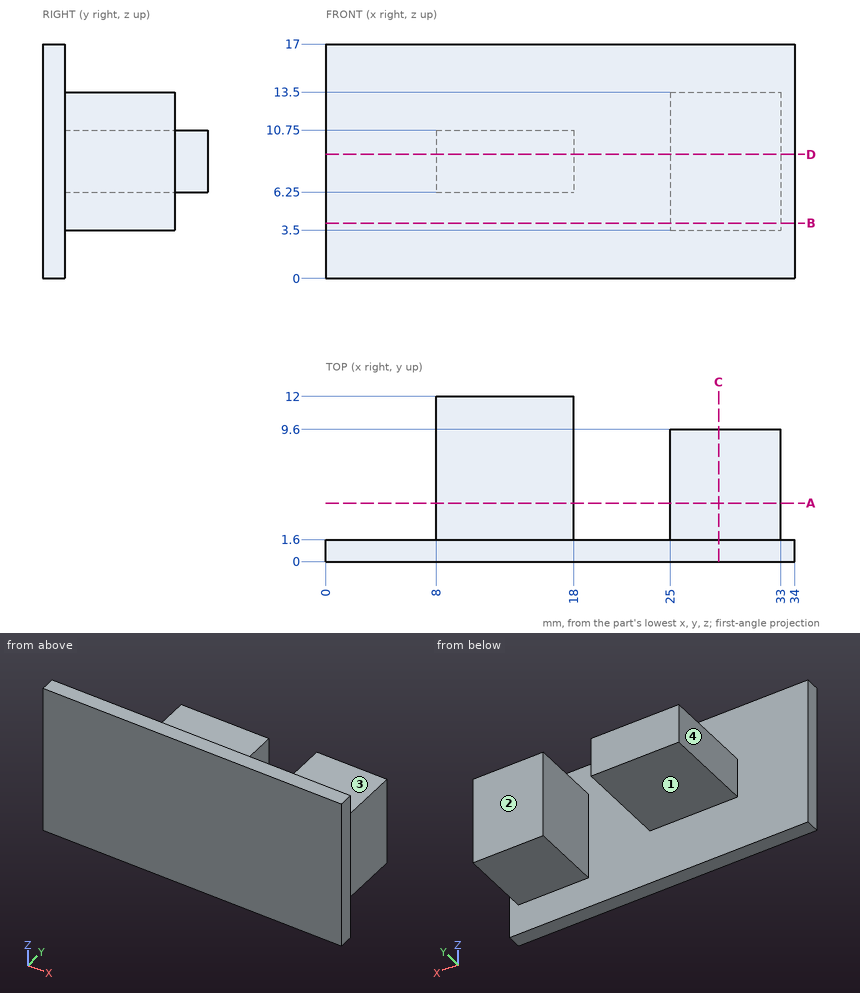
Answer from the drawing. Dimensions are ordinates in mm from the lowest x, y and z of the part. A direction names the side the tool comes from. Round coordinates to 2 decimals unless told otherwise and drop trailing zeros. Loops run counter-clockwise (first coordinate to the right, second up) from the corner with the lowest first, then second, coordinate; pieces in that order, holes last.
1) For the marked faces 1, 2, 3 and 4, determine the directions among +Z, -Z, +X, -X, +Y, -Y from which every point of the face is accessible in a straight line to the end or side of a thin tool.
Outcome:
face 1: -Z, -X, +Y
face 2: +Z, -Z, +X, +Y
face 3: +Z, +X, -X, +Y
face 4: +Z, -Z, -X, +Y
2) Given P1, Ø3.5, axis at y = 7, z = 8.5, coming from the -X side; P2, Ø3, axis at x = 12.5, z = 9, coming from the -Y side; P3, Ø6, axis at x = 4, y = 10, coming from the -Z side; P4, Ø6, axis at y = 7.5, z = 6, coming from the +X side, each flat-ended and moving along its own axis, determine where each tip first touches the part or whether it passes through.
Outcome:
P1: stops at x = 8
P2: stops at y = 0
P3: passes through
P4: stops at x = 33
3) A cutting plane is placed at A-A on y = 4.25. Determine the outline of the cut face in (x, z).
Outcome:
outline: (8, 6.25) - (18, 6.25) - (18, 10.75) - (8, 10.75) - close; (25, 3.5) - (33, 3.5) - (33, 13.5) - (25, 13.5) - close
4) A cutting plane is placed at B-B on z = 4. Determine the outline of the cut face in (x, y), plus the area to 3 significant figures.
Outcome:
outline: (0, 0) - (34, 0) - (34, 1.6) - (33, 1.6) - (33, 9.6) - (25, 9.6) - (25, 1.6) - (0, 1.6) - close
area: 118 mm2
5) A cutting plane is placed at D-D on z = 9. Determine the outline of the cut face in (x, y).
Outcome:
outline: (0, 0) - (34, 0) - (34, 1.6) - (33, 1.6) - (33, 9.6) - (25, 9.6) - (25, 1.6) - (18, 1.6) - (18, 12) - (8, 12) - (8, 1.6) - (0, 1.6) - close
6) Consider line 1 (Z direction, x = 14.5, y = 5.75); line 2 (Y direction, x = 12.5, z = 14.25); line 3 (X direction, y = 10.25, z = 7.75). Determine where each line is inside the solid, lowest interval first.
Outcome:
line 1: z = 6.25 to 10.75
line 2: y = 0 to 1.6
line 3: x = 8 to 18
7) A cutting plane is placed at C-C on x = 28.5. Determine the outline of the cut face in (y, z), plus the area to 3 significant figures.
Outcome:
outline: (0, 0) - (1.6, 0) - (1.6, 3.5) - (9.6, 3.5) - (9.6, 13.5) - (1.6, 13.5) - (1.6, 17) - (0, 17) - close
area: 107 mm2
